from build123d import *

# Parameters (mm, degrees)
ESQUISSE1_R             = 40
BOSS_EXTRU_1_DEPTH      = 0.5
ESQUISSE3_W             = 4.5
ESQUISSE3_H             = 5
ENL_V_MAT_EXTRU_1_DEPTH = 57.57075216
ENL_V_MAT_EXTRU_2_DEPTH = 57.57075216


with BuildPart() as part:
    # Esquisse1 → Boss.-Extru.1 (new body)
    with BuildSketch(Plane.XY):
        Circle(ESQUISSE1_R)
    extrude(amount=BOSS_EXTRU_1_DEPTH)

    # Esquisse3 → Enl_v. mat.-Extru.1 (cut, through all)
    with BuildSketch(Plane.XY.offset(0.5)):
        with BuildLine():
            Line((2.25, 2.5), (-2.25, 2.5))
            ThreePointArc((-2.25, 2.5), (0, 3.363406012), (2.25, 2.5))
        make_face()
        Rectangle(ESQUISSE3_W, ESQUISSE3_H)
        with BuildLine():
            ThreePointArc((2.25, -2.5), (0, -3.363406012), (-2.25, -2.5))
            Line((-2.25, -2.5), (2.25, -2.5))
        make_face()
    extrude(amount=-ENL_V_MAT_EXTRU_1_DEPTH, mode=Mode.SUBTRACT)

    # Esquisse8 → Enl_v. mat.-Extru.2 (cut, through all)
    with BuildSketch(Plane.XY.offset(0.5)):
        with BuildLine():
            Line((8.120202921, -28.880136851), (-0.775413277, -29.986633327))
            Line((-0.775413277, -29.986633327), (-1.033999584, -39.986633327))
            ThreePointArc((-1.033999584, -39.986633327), (4.952054851, -39.69228077), (10.826937228, -38.506849134))
            Line((10.826937228, -38.506849134), (8.120202921, -28.880136851))
        make_face()
    extrude(amount=-ENL_V_MAT_EXTRU_2_DEPTH, mode=Mode.SUBTRACT)


solid = part.part
CAD build for the part. Positions are in the model's coordinates, mm. A direction names the side the tool comes from. Coordinates: 2 decimals unless noted, no trailing zeros. Loops run counter-clockwise (first coordinate to the right, second up) from the corner with the lowest first, then second, coordinate; pieces in that order, holes last. Notation, with made-up numbers: (27.25, 14) - (70.25, 14) arc R16 ccw to (70.25, 38) - close; hole circle Ø8 at (11.5, -18). An arc over 180 degrees is marked (long way). Write item = value, one per line. Start each with the question number.
Q1. Cut at D-D, the plane x = -12.5. List the corners of the cut face in (y, z), then the cut area to 3 significant figures.
Q2. Drill centre lines: L1, parallel to X at y = -30.5, z = 0.4; L2, parallel to X at y = -22.5, z = 0.1; L3, parallel to Y at x = -22, z = 0.3. Where is each one in solid material? Low to high.
Q3. Which spindle directions (+Z, -Z, +X, -X, +Y, -Y) get a long thin tool onto all of the face, cutting with end or side? Do faces 1 (the flat face through (8, 1, 0.5)), 2 (the flat face through (9.493, -33.761, 0.254)). Say none if no direction does.
Q4. Cut at C-C, the plane y = 24. List the corners of the cut face in (x, z).
Q5. Cut at B-B, the plane z = 0.2. List the corners of the cut face in (x, y), then the cut area to 3 significant figures.
Q6. Cut at A-A, the plane y = 0. List the corners of the cut face in (x, z).
Computed:
q1.outline = (-38, 0) - (38, 0) - (38, 0.5) - (-38, 0.5) - close
q1.area = 38.0 mm²
q2.L1 = -25.88 to -0.79, 8.58 to 25.88
q2.L2 = -33.07 to 33.07
q2.L3 = -33.41 to 33.41
q3.face_1 = +Z, +X, -X, +Y, -Y
q3.face_2 = +Z, -Z, -Y
q4.outline = (-32, 0) - (32, 0) - (32, 0.5) - (-32, 0.5) - close
q5.outline = (-1.03, -39.99) - (-0.78, -29.99) - (8.12, -28.88) - (10.83, -38.51) arc R40 ccw (long way) to start; hole (-2.25, -2.5) arc R3.36 ccw to (2.25, -2.5) - (2.25, 2.5) arc R3.36 ccw to (-2.25, 2.5) - close
q5.area = 4,890 mm²
q6.outline = (-40, 0) - (-2.25, 0) - (-2.25, 0.5) - (-40, 0.5) - close; (2.25, 0) - (40, 0) - (40, 0.5) - (2.25, 0.5) - close
